Verification items for the finished model (mm, model axes). Face numbers are marked on the shaded views. A direction names the side the tool comes from. Give positions to 0.01 mm unless a question says otherwise; leave off trailing zeros. Write each loop counter-clockwise with the first axis right and the second up, starting at its lowest first coordinate (ties: lowest second). Pieces come first, ordered by that corner, then holes.
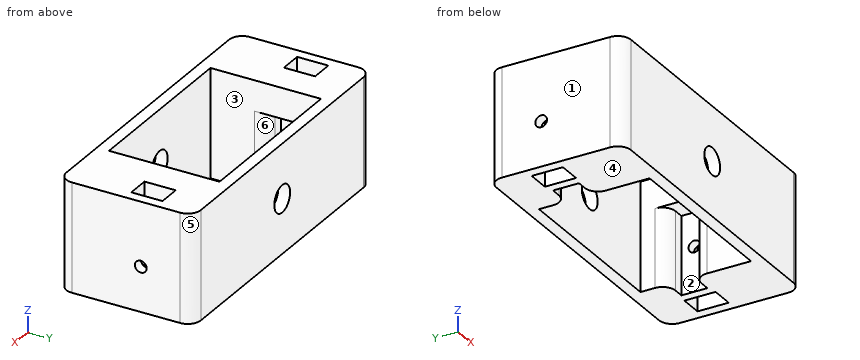
from build123d import *

# Parameters (mm, degrees)
SKETCH_1_W          = 70.2
SKETCH_1_H          = 31
EXTRUDE_1_DEPTH     = 25
SKETCH_2_W          = 40
SKETCH_2_H          = 25.5
CUT_EXTRUDE_1_DEPTH = 32
SKETCH_3_R          = 3.11
CUT_EXTRUDE_2_DEPTH = 41
SKETCH_4_W          = 5.2
SKETCH_4_H          = 7.2
CUT_EXTRUDE_3_DEPTH = 25
SKETCH_5_R          = 1.35
CUT_EXTRUDE_4_DEPTH = 122
FILLET_1_R          = 3
SKETCH_6_W          = 5.323047144
SKETCH_6_H          = 6
CUT_EXTRUDE_5_DEPTH = 18
FILLET_2_R          = 3


with BuildPart() as part:
    # 草图1 → 凸台-拉伸1 (new body)
    with BuildSketch(Plane.XY):
        Rectangle(SKETCH_1_W, SKETCH_1_H)
    extrude(amount=EXTRUDE_1_DEPTH)

    # 草图2 → 切除-拉伸1 (cut)
    with BuildSketch(Plane.XY.offset(25)):
        Rectangle(SKETCH_2_W, SKETCH_2_H)
    extrude(amount=-CUT_EXTRUDE_1_DEPTH, mode=Mode.SUBTRACT)

    # 草图3 → 切除-拉伸2 (cut)
    with BuildSketch(Plane.XZ.offset(15.5)):
        with Locations(Location((0, 12.5, 0), (0, 0, 270))):
            Circle(SKETCH_3_R)
    extrude(amount=-CUT_EXTRUDE_2_DEPTH, mode=Mode.SUBTRACT)

    # 草图4 → 切除-拉伸3 (cut)
    with BuildSketch(Plane(origin=(0, 0, 0), x_dir=(-1, 0, 0), z_dir=(0, 0, -1))):
        with Locations((30.1, 3.411480114)):
            Rectangle(SKETCH_4_W, SKETCH_4_H)
        with Locations((-30.1, 3.411480114)):
            Rectangle(SKETCH_4_W, SKETCH_4_H)
    extrude(amount=-CUT_EXTRUDE_3_DEPTH, mode=Mode.SUBTRACT)

    # 草图5 → 切除-拉伸4 (cut)
    with BuildSketch(Plane(origin=(35.1, 0, 0), x_dir=(0, 0, -1), z_dir=(1, 0, 0))):
        with Locations((-10.268877546, 3.411480114)):
            Circle(SKETCH_5_R)
    extrude(amount=-CUT_EXTRUDE_4_DEPTH, mode=Mode.SUBTRACT)

    # 圆角1
    fillet_1_edges = [part.edges().sort_by_distance(p)[0] for p in [
        (35.1, -15.5, 12.5),
        (-35.1, -15.5, 12.5),
        (-35.1, 15.5, 12.5),
        (35.1, 15.5, 12.5),
    ]]
    fillet(fillet_1_edges, radius=FILLET_1_R)

    # 草图6 → 切除-拉伸5 (cut)
    with BuildSketch(Plane(origin=(0, 0, 0), x_dir=(-1, 0, 0), z_dir=(0, 0, -1))):
        with Locations((-22.661523572, 3.411480114)):
            Rectangle(SKETCH_6_W, SKETCH_6_H)
        with Locations((22.661523572, 3.411480114)):
            Rectangle(SKETCH_6_W, SKETCH_6_H)
    extrude(amount=-CUT_EXTRUDE_5_DEPTH, mode=Mode.SUBTRACT)

    # 圆角2
    fillet_2_edges = [part.edges().sort_by_distance(p)[0] for p in [
        (20, 6.411480114, 9),
        (20, 0.411480114, 9),
        (-20, 0.411480114, 9),
        (-20, 6.411480114, 9),
    ]]
    fillet(fillet_2_edges, radius=FILLET_2_R)


solid = part.part
Item 1: Sectioned sample at B-B on y = -6. Record the cut outline in (x, z), then the cut area to 3 significant figures.
Answer key:
outline: (-35.1, 0) - (-20, 0) - (-20, 25) - (-35.1, 25) - close; (20, 0) - (35.1, 0) - (35.1, 25) - (20, 25) - close
area: 755 mm2
Item 2: Sectioned sample at C-C on z = 4. State how many separate pieces and enclosed holes the cut face has, then the cut area to 3 significant figures.
Answer key:
separate pieces: 1
enclosed holes: 3
area: 1,000 mm2
Item 3: Scan lines: line 1 along X through (y, z) = (-11, 14.75); line 2 along Y through (x, z) = (23, 7.5); line 3 along X through (y, z) = (0.5, 5.5). Record each from-to range of solid material in increasing order.
Answer key:
line 1: x = -35.1 to -20, 20 to 35.1
line 2: y = -15.5 to 0.41, 6.41 to 15.5
line 3: x = -35.1 to -32.7, -27.5 to -25.32, 25.32 to 27.5, 32.7 to 35.1
Item 4: Sectioned sample at D-D on x = 0. Record the cut outline in (y, z).
Answer key:
outline: (-15.5, 0) - (-12.75, 0) - (-12.75, 9.39) - (-15.5, 9.39) - close; (-15.5, 15.61) - (-12.75, 15.61) - (-12.75, 25) - (-15.5, 25) - close; (12.75, 0) - (15.5, 0) - (15.5, 9.39) - (12.75, 9.39) - close; (12.75, 15.61) - (15.5, 15.61) - (15.5, 25) - (12.75, 25) - close
Item 5: Release check for a two-part mould opening along X. For the marked faces 4, 5 and 6 record: released by +X, released by -X, zero draft, split by the parting line, or undercut.
Answer key:
face 4: zero draft
face 5: released by +X
face 6: undercut
Item 6: Set-up check for the marked faces 1, 2 and 3: record each of +Z, -Z, +X, -X, +Y, -Y from which the full face is reachable in a straight line by a thin tool's end or side.
Answer key:
face 1: +Z, -Z, -X, +Y, -Y
face 2: -Z
face 3: +Z, -Z
Item 7: Sectioned sample at A-A on x = 16. Record the cut outline in (y, z).
Answer key:
outline: (-15.5, 0) - (-12.75, 0) - (-12.75, 25) - (-15.5, 25) - close; (12.75, 0) - (15.5, 0) - (15.5, 25) - (12.75, 25) - close
